Can you work these out from the model? Positions are in its coordinate system, mm. Face numbers are marked on the shaded views. Give positions to 0.01 mm unless a question says otherwise; leave off trailing zeros. Loops run counter-clockwise (first coordinate to the right, second up) from the corner with the lowest first, then second, coordinate; pieces in that order, holes last. Notation, with made-up numbers: (37.25, -23.75) - (59.25, -23.75) arc R21 ccw to (59.25, 1.25) - close; hole circle Ø5 at (-31, -11). An arc over 180 degrees is marked (long way). Answer as a JSON object with one key per item and string values. Group by question number.
Item 1: Will these pins go through, and if not, where does the flat tip stop? pin 1 (6 mm diameter, centred on x = -6.94, z = -10, fed in from +Y); pin 2 (3 mm diameter, centred on x = -6.94, z = 10, fed in from -Y); pin 3 (1.8 mm diameter, centred on y = 5, z = 12.5, fed in from -X); pin 4 (3.5 mm diameter, centred on y = 5, z = -12.5, fed in from -X).
Item 2: Please list where these lines run through material, in increasing order: L1, parallel to Z at x = 3.75, y = 5; L2, parallel to Y at x = 6.75, z = -12.5; L3, parallel to Z at x = 5.5, y = 5.
Item 3: Suppose I cut it at D-D on x = -7.5. Write out the boundary of the cut face in (y, z), and give its area (3 significant figures).
Item 4: Suppose I cut it at B-B on y = 8. Write out the boundary of the cut face in (x, z), and give its area (3 significant figures).
Item 5: Thinking about a two-plate mould opening in X: for the marked faces 1, 2, 3 and 4, which applies, pulls with the +X half, pulls with the -X half, needs draft (parallel to the pull), parting line crosses it, or undercut?
Item 6: Suppose I cut it at A-A on z = 0. Write out the boundary of the cut face in (x, y).
Item 7: Suppose I cut it at C-C on x = 9.5. Write out the boundary of the cut face in (y, z).
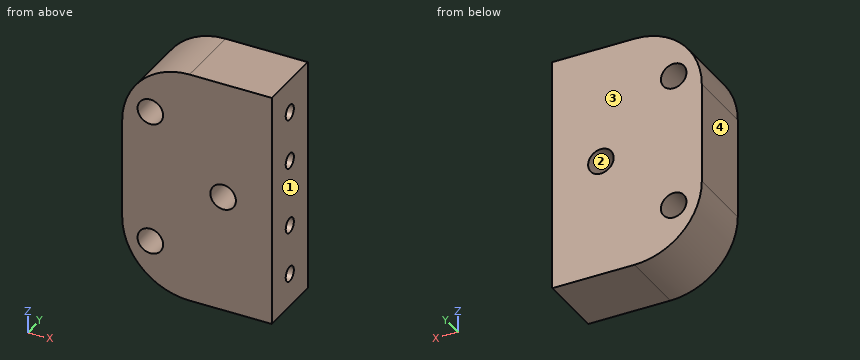
from build123d import *

# Parameters (mm, degrees)
SKETCH1_W                 = 22.2375
SKETCH1_H                 = 35
BOSS_EXTRUDE1_DEPTH       = 10
F_4_40_TAPPED_HOLE1_D     = 2.2606
F_4_40_TAPPED_HOLE1_DEPTH = 7.6
F_4_40_TAPPED_HOLE1_TIP   = 0.679152758
F_6_CLEARANCE_HOLE1_D     = 3.7973
FILLET1_R                 = 10


with BuildPart() as part:
    # Sketch1 → Boss-Extrude1 (new body)
    with BuildSketch(Plane(origin=(0, 0, 0), x_dir=(1, 0, 0), z_dir=(0, 1, 0))):
        Rectangle(SKETCH1_W, SKETCH1_H)
    extrude(amount=BOSS_EXTRUDE1_DEPTH)

    # #4-40 Tapped Hole1
    with Locations(Plane(origin=(11.11875, 0, 0), x_dir=(0, 0, -1), z_dir=(1, 0, 0))):
        with Locations((-12.5, 5), (12.5, 5), (-5, 5), (5, 5)):
            Hole(F_4_40_TAPPED_HOLE1_D / 2, depth=F_4_40_TAPPED_HOLE1_DEPTH)
            with Locations((0, 0, -(F_4_40_TAPPED_HOLE1_DEPTH + F_4_40_TAPPED_HOLE1_TIP / 2))):  # 118° drill point
                Cone(0, F_4_40_TAPPED_HOLE1_D / 2, F_4_40_TAPPED_HOLE1_TIP, mode=Mode.SUBTRACT)

    # #6 Clearance Hole1 (through all)
    with Locations(Plane(origin=(0, 10, 0), x_dir=(1, 0, 0), z_dir=(0, 1, 0))):
        with Locations((3.88125, 0), (-6.93875, 10), (-6.93875, -10)):
            Hole(F_6_CLEARANCE_HOLE1_D / 2)

    # Fillet1
    fillet1_edges = [part.edges().sort_by_distance(p)[0] for p in [
        (-11.11875, 5, 17.5),
        (-11.11875, 5, -17.5),
    ]]
    fillet(fillet1_edges, radius=FILLET1_R)


solid = part.part
Worked out:
{
 "1": {"pin 1": "stops at y = 10", "pin 2": "passes through", "pin 3": "stops at x = -10.24", "pin 4": "stops at x = -10.58"},
 "2": {"L1": "z = -17.5 to -13.63, -11.37 to -6.13, -3.87 to -1.89, 1.89 to 3.87, 6.13 to 11.37, 13.63 to 17.5", "L2": "y = 0 to 3.87, 6.13 to 10", "L3": "z = -17.5 to -13.63, -11.37 to -6.13, -3.87 to -0.99, 0.99 to 3.87, 6.13 to 11.37, 13.63 to 17.5"},
 "3": {"outline": "(0, -15.2) - (10, -15.2) - (10, -11.81) - (0, -11.81) - close; (0, -8.19) - (10, -8.19) - (10, 8.19) - (0, 8.19) - close; (0, 11.81) - (10, 11.81) - (10, 15.2) - (0, 15.2) - close", "area": "231 mm2"},
 "4": {"outline": "(-11.12, -7.5) arc R10 ccw to (-1.12, -17.5) - (11.12, -17.5) - (11.12, 17.5) - (-1.12, 17.5) arc R10 ccw to (-11.12, 7.5) - close; hole circle Ø3.8 at (-6.94, -10); hole circle Ø3.8 at (-6.94, 10); hole circle Ø3.8 at (3.88, 0)", "area": "701 mm2"},
 "5": {"face 1": "pulls with the +X half", "face 2": "undercut", "face 3": "needs draft", "face 4": "pulls with the -X half"},
 "6": {"outline": "(-11.12, 0) - (1.98, 0) - (1.98, 10) - (-11.12, 10) - close; (5.78, 0) - (11.12, 0) - (11.12, 10) - (5.78, 10) - close"},
 "7": {"outline": "(0, -17.5) - (10, -17.5) - (10, 17.5) - (0, 17.5) - close; hole circle Ø2.26 at (5, -12.5); hole circle Ø2.26 at (5, -5); hole circle Ø2.26 at (5, 5); hole circle Ø2.26 at (5, 12.5)"}
}
